```python
from build123d import *

# Parameters (mm, degrees)
F0_W     = 60
F0_H     = 30
F0_W_2   = 15.3
F0_H_2   = 5
F1_DEPTH = 6.5
F2_SIZE  = 7
F3_SIZE  = 2.5


with BuildPart() as f1:
    # F0 (on Top) → F1 (new body)
    with BuildSketch(Plane.XY):
        Rectangle(F0_W, F0_H)
        Rectangle(F0_W_2, F0_H_2, mode=Mode.SUBTRACT)
    extrude(amount=F1_DEPTH)

    # F2
    f2_edges = [f1.edges().sort_by_distance(p)[0] for p in [
        (-30, -15, 3.25),
        (30, -15, 3.25),
        (30, 15, 3.25),
        (-30, 15, 3.25),
    ]]
    chamfer(f2_edges, length=F2_SIZE)

    # F3
    f3_edges = [f1.edges().sort_by_distance(p)[0] for p in [
        (0, 15, 6.5),
        (-26.5, 11.5, 6.5),
        (-30, 0, 6.5),
        (-26.5, -11.5, 6.5),
        (0, -15, 6.5),
        (26.5, -11.5, 6.5),
        (30, 0, 6.5),
        (26.5, 11.5, 6.5),
    ]]
    chamfer(f3_edges, length=F3_SIZE)


solid = f1.part
```
Build history of the part. All positions in model axes, mm. Coordinates: 2 decimals unless noted, no trailing zeros. Order: outer loops, then holes, each group sorted by start corner. A loop starts at its lowest first (then second) coordinate and runs counter-clockwise, first axis right, second up. Notation, with made-up numbers: (52.5, 14.25) -> (64.5, 14.25) arc R18 cw to (64.5, 37.25) -> close; hole circle Ø7 at (28, 66.25). An arc over 180 degrees is marked (long way). Answer in a Markdown table with one row per item. Add a question column.
Q1. Band-saw the part on D-D, the plane x = 11.5. List the corners of the cut face in (y, z).
Q2. Band-saw the part on B-B, the plane y = -1. List the corners of the cut face in (x, z), then the cut area to 3 significant figures.
Q3. Mould opens along Y. For faces 1 (the face through (25.6, -10.7, 5.2)), 2 (the face through (0, 2.5, 3)), 3 (the face through (0, -2.5, 3)), 4 (the face through (0, 14, 5)) say: +Y half, -Y half, draft (parallel to the pull), parting line (faces both ways), or undercut.
Q4. Wall check: line 1 along X through (y, z) = (-1, 0.5); line 2 along Y through (x, z) = (2.5, 3.75); line 3 along X through (y, z) = (10.5, 3.5). Give the ranges that are in metal, low to high. Write a range as [from, to].
Q5. Band-saw the part on C-C, the plane z = 0.75. List the corners of the cut face in (x, y).
Q6. Band-saw the part on A-A, the plane x = 4. List the corners of the cut face in (y, z), then the cut area to 3 significant figures.
Answers follow:
| question | item | result |
|---|---|---|
| 1 | outline | (-15, 0) -> (15, 0) -> (15, 4) -> (12.5, 6.5) -> (-12.5, 6.5) -> (-15, 4) -> close |
| 2 | outline | (-30, 0) -> (-7.65, 0) -> (-7.65, 6.5) -> (-27.5, 6.5) -> (-30, 4) -> close; (7.65, 0) -> (30, 0) -> (30, 4) -> (27.5, 6.5) -> (7.65, 6.5) -> close |
| 2 | area | 284 mm^2 |
| 3 | face 1 | -Y half |
| 3 | face 2 | undercut |
| 3 | face 3 | undercut |
| 3 | face 4 | +Y half |
| 4 | line 1 | [-30, -7.65], [7.65, 30] |
| 4 | line 2 | [-15, -2.5], [2.5, 15] |
| 4 | line 3 | [-27.5, 27.5] |
| 5 | outline | (-30, -8) -> (-23, -15) -> (23, -15) -> (30, -8) -> (30, 8) -> (23, 15) -> (-23, 15) -> (-30, 8) -> close; hole (-7.65, -2.5) -> (7.65, -2.5) -> (7.65, 2.5) -> (-7.65, 2.5) -> close |
| 6 | outline | (-15, 0) -> (-2.5, 0) -> (-2.5, 6.5) -> (-12.5, 6.5) -> (-15, 4) -> close; (2.5, 0) -> (15, 0) -> (15, 4) -> (12.5, 6.5) -> (2.5, 6.5) -> close |
| 6 | area | 156 mm^2 |
